Model file for the job. Use its own axes, mm. A direction names the side the tool comes from. Coordinates: 2 decimals unless noted, no trailing zeros. Write each loop counter-clockwise with the first axis right and the second up, starting at its lowest first coordinate (ties: lowest second). Pieces come first, ordered by that corner, then holes. Notation, with made-up numbers: M 33.25,79 L 91.25,79 A11 cw 91.25,83 Z; hole C 58.5,-24.75 d10. An arc over 180 degrees is marked long. Put each result on its own line as item: value. Start each with the question number.
Q1. Which spindle directions (+Z, -Z, +X, -X, +Y, -Y) get a long thin tool onto all of the face, cutting with end or side? Do faces 1 (the flat face through (45, -20.709, 9)), 2 (the flat face through (49.356, -17, -16)), 3 (the flat face through (52.531, -24, -3)), 4 (the cylindrical face through (44.94, -38.52, 12.67)). Say none if no direction does.
Q2. Cut at C-C (y = -4.5). Write the cut outline in (x, z) (3 decimals).
Q3. Pull direction Z, two halves, no side cores. Call faces 5 (the cylindrical face through (43.006, -16.828, 19.157)), 6 (the cylindrical face through (-3.676, -1.565, -35.577)), 7 (the flat face through (3.175, -17, -16)), 8 (the flat face through (50.966, -25.375, -22.745)): pulls with the +Z half, pulls with the -Z half, needs draft (parallel to the pull), parting line crosses it, or undercut.
Q4. Drill centre lines: line 1 along X through (y, z) = (-7.5, -2.5) (3 decimals); line 2 along Y through (x, z) = (45, 3.5); line 3 along Z through (x, y) = (24, -2) (3 decimals). Where is each one in solid material? Low to high.
Q5. Cut at D-D (z = -23.5). Write the cut outline in (x, y) (1 decimal).
Q6. Drop flat-ended pins along their axis: pin 1 (2 mm diameter, centred on x = 21.5, y = -4.5, fed in from -Z); pin 2 (6 mm diameter, centred on y = -21, z = -9, fed in from -X); pin 3 (8 mm diameter, centred on y = -35.5, z = 14, fed in from +X); pin 4 (2.5 mm diameter, centred on x = -3.97, z = -0.79, fed in from -Y). Give the stop position or say it passes through.
Q7. Cut at B-B (x = 36). Write the cut outline in (y, z) (1 decimal), then the cut area to 3 significant figures.
```python
from build123d import *

# Parameters (mm, degrees)
F0_W         = 52.5309846
F0_H         = 44.9404867
F0_R         = 1.5
F0_R_2       = 11.2530001
F1_DEPTH     = 3.175
F2_W         = 3.175
F2_H         = 44.9404867
F3_DEPTH     = 41.774999
F4_W         = 7.9375
F4_H         = 3.175
F5_DEPTH     = 44.949999
F6_R         = 3.96875
F7_R         = 2.2479
F8_DEPTH     = 3.175
F10_DEPTH    = 52.5309846
F12_DEPTH    = 19.2659
F14_DEPTH    = 10.7654979
F15_T1_DEPTH = 47.0239979
F16_R        = 2
F17_DEPTH    = 134
F18_R        = 7.9375
F19_DEPTH    = 25.4


# Not quite as in the source:
# - a fillet or chamfer that OpenCascade refuses, or shapes differently, is made with other operations: its cross-section is extruded or revolved along the edge and cut away or added
# - an extrude ends at something that could not be found from the text; its depth is read off the source's solid
# - a feature names something its author has since deleted; it is built from what else it names


with BuildPart() as f1:
    # F0 (on Top) → F1 (new body)
    with BuildSketch(Plane.XY):
        with Locations((26.2654923, -22.47024335)):
            Rectangle(F0_W, F0_H)
        with Locations((10.7654979, -38.5904867)):
            Circle(F0_R, mode=Mode.SUBTRACT)
        with Locations((26.2654923, -23.0904923)):
            Circle(F0_R_2, mode=Mode.SUBTRACT)
        with Locations((41.7654867, -38.5904867)):
            Circle(F0_R, mode=Mode.SUBTRACT)
        with Locations((10.7654979, -7.5904979)):
            Circle(F0_R, mode=Mode.SUBTRACT)
        with Locations((41.7654867, -7.5904979)):
            Circle(F0_R, mode=Mode.SUBTRACT)
    extrude(amount=F1_DEPTH)

    # F2 (on face) → F3 (join)
    with BuildSketch(Plane(origin=(0, 0, 0), x_dir=(1, 0, 0), z_dir=(0, 0, -1))):
        with Locations((1.5875, 22.47024335)):
            Rectangle(F2_W, F2_H)
        with Locations((50.9434846, 22.47024335)):
            Rectangle(F2_W, F2_H)
    extrude(amount=F3_DEPTH)

    # F4 (on face) → F5 (join, through all)
    with BuildSketch(Plane(origin=(0, 0, -41.774999), x_dir=(1, 0, 0), z_dir=(0, 0, -1))):
        with Locations((-3.96875, 1.5875)):
            Rectangle(F4_W, F4_H)
        with Locations((56.4997346, 1.5875)):
            Rectangle(F4_W, F4_H)
    extrude(amount=-F5_DEPTH)

    # F6
    f6_edges = [f1.edges().sort_by_distance(p)[0] for p in [
        (60.468485, -1.5875, -41.774999),
        (60.468485, -1.5875, 3.175),
        (-7.9375, -1.5875, 3.175),
        (-7.9375, -1.5875, -41.774999),
    ]]
    fillet(f6_edges, radius=F6_R)

    # F7 (on face) → F8 (cut, through all)
    with BuildSketch(Plane(origin=(0, 0, 0), x_dir=(-1, 0, 0), z_dir=(0, 1, 0))):
        with Locations((3.96875, -37.806249)):
            Circle(F7_R)
        with Locations((3.96875, -0.79375)):
            Circle(F7_R)
        with Locations((-56.4997346, -0.79375)):
            Circle(F7_R)
        with Locations((-56.4997346, -37.806249)):
            Circle(F7_R)
    extrude(amount=-F8_DEPTH, mode=Mode.SUBTRACT)

    # F9 (on face) → F10 (cut, through all)
    with BuildSketch(Plane.YZ.offset(52.5309846)):
        Polygon((-44.9404867, -3.175), (-44.9404867, -41.774999), (-6.35, -41.774999), align=None)
    extrude(amount=-F10_DEPTH, mode=Mode.SUBTRACT)

    # F11 (on face) → F12 (join)
    with BuildSketch(Plane.XY.offset(3.175)):
        with BuildLine():
            Line((41.7654867, -44.9404867), (52.5309846, -44.9404867))
            Line((52.5309846, -44.9404867), (52.5309846, -30.4370867))
            Line((52.5309846, -30.4370867), (41.7654867, -30.4370867))
            Line((41.7654867, -30.4370867), (41.7654867, -35.4154867))
            ThreePointArc((41.7654867, -35.4154867), (44.9404867, -38.5904867), (41.7654867, -41.7654867))
            Line((41.7654867, -41.7654867), (41.7654867, -44.9404867))
        make_face()
        with BuildLine():
            Line((52.5309846, -20.7092423), (52.5309846, -12.7717423))
            Line((52.5309846, -12.7717423), (30.7547472146, -12.7717423))
            ThreePointArc((30.7547472146, -12.7717423), (34.966988133, -15.9550889113), (37.2636584966, -20.7092423))
            Line((37.2636584966, -20.7092423), (52.5309846, -20.7092423))
        make_face()
    extrude(amount=F12_DEPTH)

    # F13 (on face) → F14 (cut, through all)
    with BuildSketch(Plane.YZ.offset(52.5309846)):
        with BuildLine():
            Line((-40.0700367, 15.1892), (-37.6887867, 15.1892))
            Line((-37.6887867, 15.1892), (-37.6887867, 12.80795))
            ThreePointArc((-37.6887867, 12.80795), (-36.0049886773, 13.5054019773), (-35.3075367, 15.1892))
            ThreePointArc((-35.3075367, 15.1892), (-37.6887867, 17.57045), (-40.0700367, 15.1892))
        make_face()
        with BuildLine():
            Line((-37.6887867, 12.80795), (-37.6887867, 15.1892))
            Line((-37.6887867, 15.1892), (-40.0700367, 15.1892))
            ThreePointArc((-40.0700367, 15.1892), (-39.3725847227, 13.5054019773), (-37.6887867, 12.80795))
        make_face()
    extrude(amount=-F14_DEPTH, mode=Mode.SUBTRACT)

    # F15: fillet of radius 7.2517 on 2 edges, made by hand

    # F15_s2 → F15_t1 (cut)
    with BuildSketch(Plane.YZ.offset(23.6362367)):
        with BuildLine():
            ThreePointArc((-44.9404867, 15.1892), (-42.8165129451, 20.3169262451), (-37.6887867, 22.4409))
            Line((-37.6887867, 22.4409), (-44.9404867, 22.4409))
            Line((-44.9404867, 22.4409), (-44.9404867, 15.1892))
        make_face()
        with BuildLine():
            ThreePointArc((-30.4370867, 15.1892), (-32.5610604549, 20.3169262451), (-37.6887867, 22.4409))
            Line((-37.6887867, 22.4409), (-30.4370867, 22.4409))
            Line((-30.4370867, 22.4409), (-30.4370867, 15.1892))
        make_face()
    extrude(amount=F15_T1_DEPTH, mode=Mode.SUBTRACT)

    # F16 (on face) → F17 (cut, through all)
    with BuildSketch(Plane.YZ.offset(52.5309846)):
        with BuildLine():
            Line((-12.7717423, 22.4409), (-20.7092423, 22.4409))
            Line((-20.7092423, 22.4409), (-20.7092423, 15.1892))
            ThreePointArc((-20.7092423, 15.1892), (-16.7404923, 19.15795), (-12.7717423, 15.1892))
            Line((-12.7717423, 15.1892), (-12.7717423, 22.4409))
        make_face()
        with Locations((-16.7404923, 15.1892)):
            Circle(F16_R)
    extrude(amount=-F17_DEPTH, mode=Mode.SUBTRACT)

    # F18 (on face) → F19 (cut)
    with BuildSketch(Plane.XY.offset(3.175)):
        with Locations((26.2654923, -10.3904923)):
            Circle(F18_R)
    extrude(amount=F19_DEPTH, mode=Mode.SUBTRACT)


solid = f1.part
```
Computed values:
1. face 1: +Z, +X, -X
1. face 2: -Z, +Y, -Y
1. face 3: +Z, -Z, +X, -Y
1. face 4: +Z, -X
2. outline: M 0,-41.775 L 3.175,-41.775 L 3.175,0 L 49.356,0 L 49.356,-41.775 L 52.531,-41.775 L 52.531,3.175 L 0,3.175 Z
3. face 5: pulls with the +Z half
3. face 6: undercut
3. face 7: needs draft
3. face 8: pulls with the -Z half
4. line 1: 0 to 3.175, 49.356 to 52.531
4. line 2: -44.94 to -30.44, -20.71 to -12.77
4. line 3: 0 to 3.175
5. outline: M -7.9,-3.2 L 0,-3.2 L 0,-24.6 L 3.2,-24.6 L 3.2,0 L -7.9,0 Z; M 49.4,-24.6 L 52.5,-24.6 L 52.5,-3.2 L 60.5,-3.2 L 60.5,0 L 49.4,0 Z
6. pin 1: z = 0
6. pin 2: x = 0
6. pin 3: x = 52.53
6. pin 4: through
7. outline: M -44.9,0 L -28.7,0 L -28.7,3.2 L -44.9,3.2 Z; M -17.4,0 L 0,0 L 0,3.2 L -12.8,3.2 L -12.8,15.2 A4 ccw -17.4,19.1 L -17.4,17.1 A2 cw long -17.4,13.3 Z
7. area: 169 mm2
